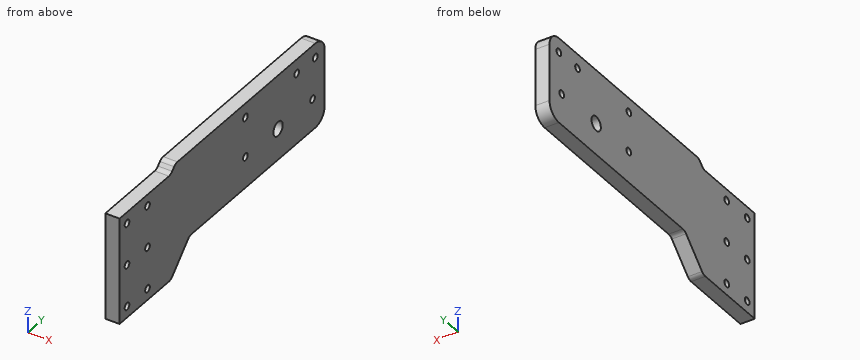
```python
from build123d import *

# Parameters (mm, degrees)
SKETCH1_R           = 2.5
SKETCH1_R_2         = 5
BOSS_EXTRUDE1_DEPTH = 10


with BuildPart() as part:
    # Sketch1 → Boss-Extrude1 (new body)
    with BuildSketch(Plane(origin=(0, 0, 0), x_dir=(0, 0, -1), z_dir=(1, 0, 0))):
        with BuildLine():
            Line((0, 0), (75, 0))
            Line((75, 0), (75, 52.928932188))
            ThreePointArc((75, 52.928932188), (74.619397663, 54.84234935), (73.535533906, 56.464466094))
            Line((73.535533906, 56.464466094), (56.464466094, 73.535533906))
            ThreePointArc((56.464466094, 73.535533906), (55.380602337, 75.15765065), (55, 77.071067812))
            Line((55, 77.071067812), (55, 210))
            ThreePointArc((55, 210), (52.071067812, 217.071067812), (45, 220))
            Line((45, 220), (5, 220))
            ThreePointArc((5, 220), (-2.071067812, 217.071067812), (-5, 210))
            Line((-5, 210), (-5, 62.071067812))
            ThreePointArc((-5, 62.071067812), (-4.619397663, 60.15765065), (-3.535533906, 58.535533906))
            Line((-3.535533906, 58.535533906), (-1.464466094, 56.464466094))
            ThreePointArc((-1.464466094, 56.464466094), (-0.380602337, 54.84234935), (0, 52.928932188))
            Line((0, 52.928932188), (0, 0))
        make_face()
        with Locations((5, 210)):
            Circle(SKETCH1_R, mode=Mode.SUBTRACT)
        with Locations((5, 190)):
            Circle(SKETCH1_R, mode=Mode.SUBTRACT)
        with Locations((33, 207)):
            Circle(SKETCH1_R, mode=Mode.SUBTRACT)
        with Locations((5, 135)):
            Circle(SKETCH1_R, mode=Mode.SUBTRACT)
        with Locations((33, 135)):
            Circle(SKETCH1_R, mode=Mode.SUBTRACT)
        with Locations((8, 30)):
            Circle(SKETCH1_R, mode=Mode.SUBTRACT)
        with Locations((8, 8)):
            Circle(SKETCH1_R, mode=Mode.SUBTRACT)
        with Locations((37.5, 8)):
            Circle(SKETCH1_R, mode=Mode.SUBTRACT)
        with Locations((37.5, 30)):
            Circle(SKETCH1_R, mode=Mode.SUBTRACT)
        with Locations((67, 30)):
            Circle(SKETCH1_R, mode=Mode.SUBTRACT)
        with Locations((67, 8)):
            Circle(SKETCH1_R, mode=Mode.SUBTRACT)
        with Locations((33, 170)):
            Circle(SKETCH1_R_2, mode=Mode.SUBTRACT)
    extrude(amount=BOSS_EXTRUDE1_DEPTH)


solid = part.part
```
For this review, take the finished solid that the model builds, in its own axes (mm). Round coordinates to 2 decimals unless told otherwise and drop trailing zeros. Order: outer loops, then holes, each group sorted by start corner. A loop starts at its lowest first (then second) coordinate and runs counter-clockwise, first axis right, second up. Notation, with made-up numbers: (-39, 65) -> (-29, 65) arc R32 ccw to (-29, 96) -> close; hole circle Ø2 at (-38, 51.25). An arc over 180 degrees is marked (long way). Use a Markdown table: item, result.
Item 1: Take a section at C-C (x = 3.25). State how many separate pieces and enclosed holes the cut face has, plus the area to 3 significant figures.
Resolved:
| item | result |
|---|---|
| separate pieces | 1 |
| enclosed holes | 12 |
| area | 13,900 mm² |
Item 2: Take a section at D-D (z = -33). State the section outline as (x, y) points.
Resolved:
| item | result |
|---|---|
| outline | (0, 0) -> (10, 0) -> (10, 132.5) -> (0, 132.5) -> close; (0, 137.5) -> (10, 137.5) -> (10, 165) -> (0, 165) -> close; (0, 175) -> (10, 175) -> (10, 204.5) -> (0, 204.5) -> close; (0, 209.5) -> (10, 209.5) -> (10, 220) -> (0, 220) -> close |
Item 3: Take a section at B-B (z = -67). State the section outline as (x, y) points.
Resolved:
| item | result |
|---|---|
| outline | (0, 0) -> (10, 0) -> (10, 5.5) -> (0, 5.5) -> close; (0, 10.5) -> (10, 10.5) -> (10, 27.5) -> (0, 27.5) -> close; (0, 32.5) -> (10, 32.5) -> (10, 63) -> (0, 63) -> close |
Item 4: For line 1 along Z through (x, y) = (3, 135); line 2 along Y through (x, z) = (7.75, -5); line 3 along Y through (x, z) = (4, -8), list the stretches that pass through material, from the lowest coordinate up. Write a range as [from, to].
Resolved:
| item | result |
|---|---|
| line 1 | z = [-55, -35.5], [-30.5, -7.5], [-2.5, 5] |
| line 2 | y = [0, 132.5], [137.5, 187.5], [192.5, 207.5], [212.5, 220] |
| line 3 | y = [0, 5.5], [10.5, 27.5], [32.5, 220] |
Item 5: For pin 1 (6 mm diameter, centred on x = 8.5, y = 70.5, fed in from -Z); pin 2 (6 mm diameter, centred on x = 7.5, y = 70, fed in from -Z); pin 3 (3 mm diameter, centred on x = 3.5, y = 70, fed in from -Z), all flat-tipped, find the tip position at first contact; note any pin that passes through.
Resolved:
| item | result |
|---|---|
| pin 1 | stops at z = -62.5 |
| pin 2 | stops at z = -63 |
| pin 3 | stops at z = -61.5 |
Item 6: Take a section at A-A (y = 170). State the section outline as (x, z) points, plus the area to 3 significant figures.
Resolved:
| item | result |
|---|---|
| outline | (0, -55) -> (10, -55) -> (10, -38) -> (0, -38) -> close; (0, -28) -> (10, -28) -> (10, 5) -> (0, 5) -> close |
| area | 500 mm² |
